Design review of the part shown in the three views and the two pictorial views. Dimensions are in mm from the part's minimum x, y and z. A direction names the side the tool comes from. Coordinates: 2 decimals unless noted, no trailing zeros. Order: outer loops, then holes, each group sorted by start corner. A loop starts at its lowest first (then second) coordinate and runs counter-clockwise, first axis right, second up. Notation, with made-up numbers: M 81,73 L 117,73 A33 cw 117,104 Z; hole C 51,67 d11. An arc over 180 degrees is marked long. Use CSV: the item, a comma, the result in double quotes.
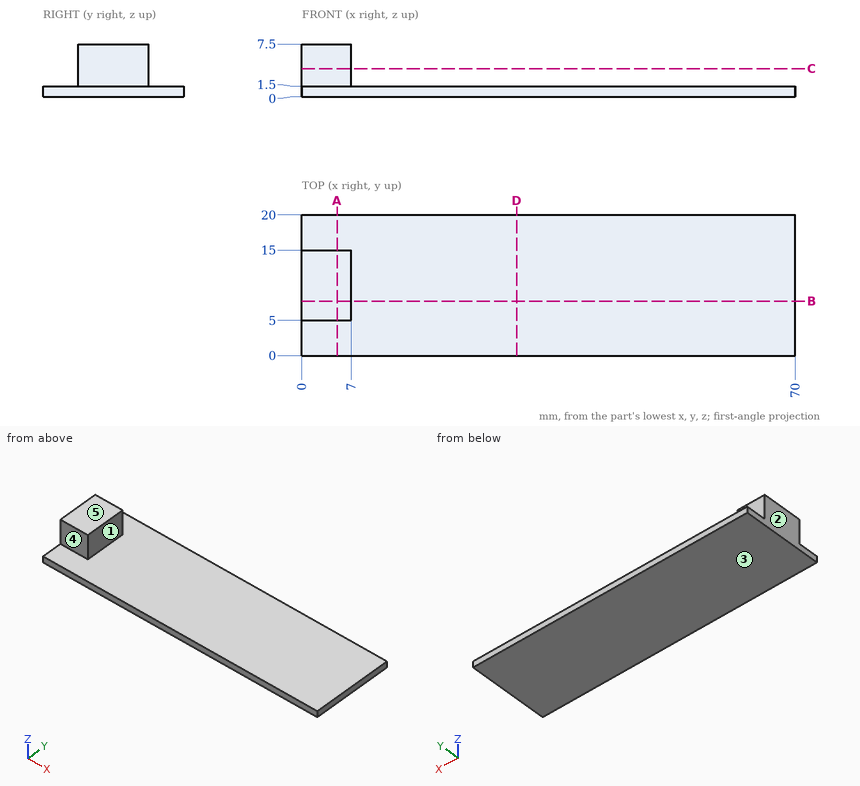
(1) Add section D-D on x = 30.5. State the section outline as (y, z) points, and give its area (3 significant figures).
The answers:
outline,"M 0,0 L 20,0 L 20,1.5 L 0,1.5 Z"
area,"30.0 mm2"
(2) Add section C-C on z = 4. State the section outline as (x, y) points, and give its area (3 significant figures).
The answers:
outline,"M 0,5 L 7,5 L 7,15 L 0,15 Z"
area,"70.0 mm2"
(3) Clearance check with flat-ended pins moving along their axes: P1, Ø1.8, axis at x = 4.5, z = 6, coming from the -Y side; P2, Ø1.8, axis at y = 9.5, z = 3.5, coming from the +X side; P3, Ø1.8, axis at x = 2.5, z = 5, coming from the +Y side. State where each tip first meets the part, or that it passes through.
The answers:
P1,"stops at y = 5"
P2,"stops at x = 7"
P3,"stops at y = 15"
(4) The part is to be moulded in two halves that separate along X. For the marked faces 1, 2 and 3, say which applies: pulls with the +X half, pulls with the -X half, needs draft (parallel to the pull), parting line crosses it, or undercut.
The answers:
face 1,"pulls with the +X half"
face 2,"pulls with the -X half"
face 3,"needs draft"
(5) Wall thickness on probe 1 along Z at (x, y) = (50, 9.5); probe 2 along X at (y, z) = (6.25, 1.75): over which ranges is each line inside the solid? List them lowest first.
The answers:
probe 1,"z = 0 to 1.5"
probe 2,"x = 0 to 7"
(6) Add section B-B on y = 7.75. State the section outline as (x, z) points.
The answers:
outline,"M 0,0 L 70,0 L 70,1.5 L 7,1.5 L 7,7.5 L 0,7.5 Z"
(7) Add section A-A on x = 5. State the section outline as (y, z) points.
The answers:
outline,"M 0,0 L 20,0 L 20,1.5 L 15,1.5 L 15,7.5 L 5,7.5 L 5,1.5 L 0,1.5 Z"
(8) For the marked faces 4 and 5, list the 3-axis set-ups (+Z, -Z, +X, -X, +Y, -Y) from which the entire face can be reached by the end or side of a thin tool; tool diameter is ignored.
The answers:
face 4,"+Z, +X, -X, -Y"
face 5,"+Z, +X, -X, +Y, -Y"
